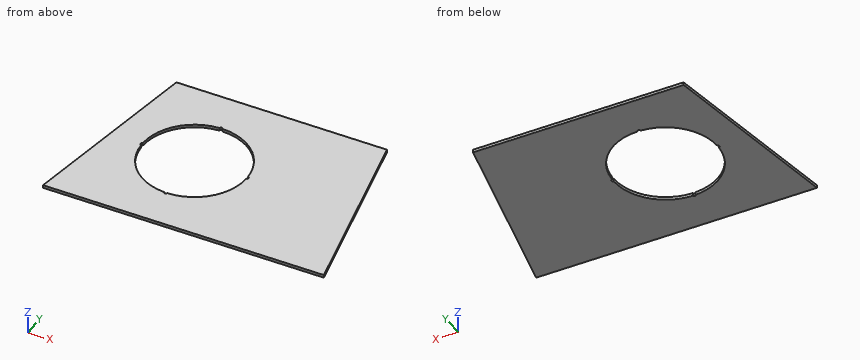
from build123d import *

# Parameters (mm, degrees)
F1_DEPTH = 3.175
F3_D     = 3.175
F3_DEPTH = 17.4625


with BuildPart() as f1:
    # F0 (on Top) → F1 (new body)
    with BuildSketch(Plane.XY):
        Polygon((-108.327691, 182.628707), (-146.427691, -20.571293), (158.372309, -20.571293), (120.272309, 182.628707), (5.972309, 182.628707), align=None)
        with BuildLine():
            ThreePointArc((-35.302691, 138.178707), (5.108462, 121.439859), (21.847309, 81.028707))
            ThreePointArc((21.847309, 81.028707), (5.108462, 40.617554), (-35.302691, 23.878707))
            ThreePointArc((-35.302691, 23.878707), (-75.713844, 40.617554), (-92.452691, 81.028707))
            ThreePointArc((-92.452691, 81.028707), (-75.713844, 121.439859), (-35.302691, 138.178707))
        make_face(mode=Mode.SUBTRACT)
    extrude(amount=F1_DEPTH)

    # F3
    with Locations(Plane.XY.offset(3.175)):
        with Locations((-36.544064, 138.165223), (21.847309, 81.028707), (-36.544064, 23.89219), (-92.452691, 81.028707)):
            Hole(F3_D / 2, depth=F3_DEPTH)


solid = f1.part
Can you work these out from the model? Positions are in its coordinate system, mm. Give positions to 0.01 mm unless a question says otherwise; leave off trailing zeros. Order: outer loops, then holes, each group sorted by start corner. A loop starts at its lowest first (then second) coordinate and runs counter-clockwise, first axis right, second up. Notation, with made-up numbers: M 14.25,-7 L 71.25,-7 A26 cw 71.25,23 Z; hole C -25,57 d11. An arc over 180 degrees is marked long. Use one line per item in the form item = value.
Item 1: If we section it at B-B, the plane y = 113.5: Write out the boundary of the cut face in (x, z) (3 decimals), and give its area (3 significant figures).
Values follow:
outline = M -121.289,0 L -82.332,0 L -82.332,3.175 L -121.289,3.175 Z; M 11.726,0 L 133.234,0 L 133.234,3.175 L 11.726,3.175 Z
area = 509 mm^2
Item 2: Will this pin go through, and if not, where does the flat tip stop? pin 1 Ø1.5 at (y, z) = (151, 1) entering from +X.
Values follow:
pin_1 = 126.34
Item 3: If we section it at D-D, the plane y = 154: Write out the boundary of the cut face in (x, z) (3 decimals), and give its area (3 significant figures).
Values follow:
outline = M -113.696,0 L 125.64,0 L 125.64,3.175 L -113.696,3.175 Z
area = 760 mm^2
Item 4: If we section it at C-C, the plane x = -53: Write out the boundary of the cut face in (y, z) (3 decimals), and give its area (3 significant figures).
Values follow:
outline = M -20.571,0 L 26.688,0 L 26.688,3.175 L -20.571,3.175 Z; M 135.37,0 L 182.629,0 L 182.629,3.175 L 135.37,3.175 Z
area = 300 mm^2
Item 5: If I drill on line 1 along Y through (x, z) = (-37, 1.8); line 2 along X through (y, z) = (82, 2.5); line 3 along X through (y, z) = (100.5, 2.65), over which ranges is the centre line in solid material (lowest first)? Write a range as [from, to].
Values follow:
line_1 = [-20.57, 22.37], [139.69, 182.63]
line_2 = [-127.2, -93.71], [23.1, 139.14]
line_3 = [-123.73, -89.03], [18.43, 135.67]
